Design review of the part built by this model. Coordinates are the model's own, in mm. Face numbers are marked on the shaded views. A direction names the side the tool comes from. Coordinates: 2 decimals unless noted, no trailing zeros. Order: outer loops, then holes, each group sorted by start corner. A loop starts at its lowest first (then second) coordinate and runs counter-clockwise, first axis right, second up. Notation, with made-up numbers: (17, 73.5) - (75, 73.5) arc R20 cw to (75, 93.5) - close; hole circle Ø1 at (80.5, 21). An arc over 180 degrees is marked (long way). Write item = value, one per line. Start each with the question number.
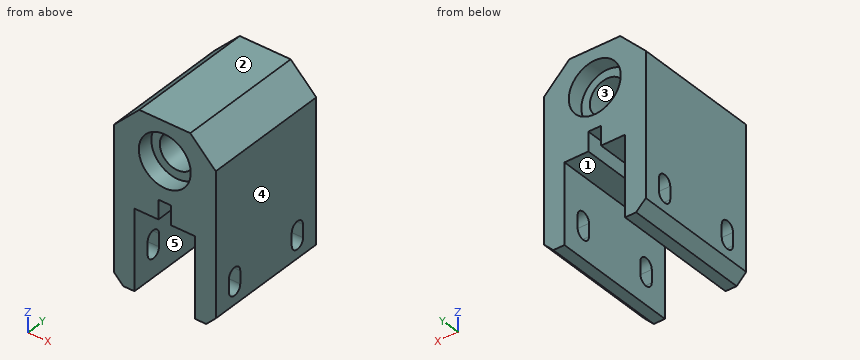
```python
from build123d import *

# Parameters (mm, degrees)
SKETCH1_R           = 5.5
BOSS_EXTRUDE1_DEPTH = 20
SKETCH2_R           = 8.15
CUT_EXTRUDE1_DEPTH  = 5
CUT_EXTRUDE2_DEPTH  = 58.586890869


with BuildPart() as part:
    # Sketch1 → Boss-Extrude1 (new, symmetric)
    with BuildSketch(Plane(origin=(0, 0, 0), x_dir=(1, 0, 0), z_dir=(0, 1, 0))):
        Polygon((-9.5, 43.5), (-9.5, 18.5), (-2, 18.5), (-2, 12.5), (2, 12.5), (2, 18.5), (9.5, 18.5), (9.5, 43.5), (13, 43.5), (16, 40.5), (16, -4), (8, -12), (-8, -12), (-16, -4), (-16, 40.5), (-13, 43.5), align=None)
        with Locations(Location((0, 0, 0), (0, 0, 270))):
            Circle(SKETCH1_R, mode=Mode.SUBTRACT)
    extrude(amount=BOSS_EXTRUDE1_DEPTH, both=True)

    # Sketch2 → Cut-Extrude1 (cut)
    with BuildSketch(Plane(origin=(0, 20, 0), x_dir=(1, 0, 0), z_dir=(0, 1, 0))):
        with Locations(Location((0, 0, 0), (0, 0, 270))):
            Circle(SKETCH2_R)
    cut_extrude1 = extrude(amount=-CUT_EXTRUDE1_DEPTH, mode=Mode.SUBTRACT)

    # Mirror1: Cut-Extrude1 across plane
    add(cut_extrude1.mirror(Plane.ZX), mode=Mode.SUBTRACT)

    # Sketch3 → Cut-Extrude2 (cut, through all)
    with BuildSketch(Plane(origin=(16, 0, 0), x_dir=(0, 0, -1), z_dir=(1, 0, 0))):
        with BuildLine():
            Line((35.5, 10.25), (31.5, 10.25))
            ThreePointArc((31.5, 10.25), (29.25, 12.5), (31.5, 14.75))
            Line((31.5, 14.75), (35.5, 14.75))
            ThreePointArc((35.5, 14.75), (37.75, 12.5), (35.5, 10.25))
        make_face()
        with BuildLine():
            Line((35.5, -14.75), (31.5, -14.75))
            ThreePointArc((31.5, -14.75), (29.25, -12.5), (31.5, -10.25))
            Line((31.5, -10.25), (35.5, -10.25))
            ThreePointArc((35.5, -10.25), (37.75, -12.5), (35.5, -14.75))
        make_face()
    extrude(amount=-CUT_EXTRUDE2_DEPTH, mode=Mode.SUBTRACT)


solid = part.part
```
Item 1: Add section B-B on z = -21. Give the boundary of the cut face in (x, y).
Item 2: Mouldability with a two-part tool opening along Z and no side actions: class the marked faces 1, 2 and 3 as +Z half, -Z half, draft (parallel to the pull), parting line (faces both ways), or undercut.
Item 3: For line 1 (X direction, y = -18.7, z = 0); line 2 (X direction, y = 4.25, z = 0); line 3 (Z direction, x = -12, y = 16), list the stretches that pass through material, from the lowest coordinate up.
Item 4: Add section A-A on y = 12.5. Give the boundary of the cut face in (x, z).
Item 5: Add section D-D on x = 12. Give the boundary of the cut face in (y, z).
Item 6: Add section C-C on x = 0. Give the boundary of the cut face in (y, z), plus the area to 3 significant figures.
Item 7: For P1, Ø6, axis at x = -7, y = -8, coming from the -Z side; P2, Ø5, axis at x = 6.5, y = 5, coming from the -Z side; P3, Ø2, axis at x = 0, y = -10, coming from the -Z side, all flat-tipped, find the tip position at first contact; note any pin that passes through.
Item 8: For the marked faces 4 and 5, list the 3-axis set-ups (+Z, -Z, +X, -X, +Y, -Y) from which the entire face can be reached by the end or side of a thin tool; tool diameter is ignored.
Worked out:
q1.outline = (-16, -20) - (-9.5, -20) - (-9.5, 20) - (-16, 20) - close; (9.5, -20) - (16, -20) - (16, 20) - (9.5, 20) - close
q2.face_1 = -Z half
q2.face_2 = +Z half
q2.face_3 = undercut
q3.line_1 = -16 to -8.15, 8.15 to 16
q3.line_2 = -16 to -5.5, 5.5 to 16
q3.line_3 = -43.5 to 8
q4.outline = (-16, -40.5) - (-13, -43.5) - (-9.5, -43.5) - (-9.5, -37.75) - (-16, -37.75) - close; (-16, -29.25) - (-9.5, -29.25) - (-9.5, -18.5) - (-2, -18.5) - (-2, -12.5) - (2, -12.5) - (2, -18.5) - (9.5, -18.5) - (9.5, -29.25) - (16, -29.25) - (16, 4) - (8, 12) - (-8, 12) - (-16, 4) - close; (9.5, -43.5) - (13, -43.5) - (16, -40.5) - (16, -37.75) - (9.5, -37.75) - close; hole circle Ø11 at (0, 0)
q5.outline = (-20, -43.5) - (20, -43.5) - (20, 8) - (-20, 8) - close; hole (-14.75, -35.5) arc R2.25 ccw to (-10.25, -35.5) - (-10.25, -31.5) arc R2.25 ccw to (-14.75, -31.5) - close; hole (10.25, -35.5) arc R2.25 ccw to (14.75, -35.5) - (14.75, -31.5) arc R2.25 ccw to (10.25, -31.5) - close
q6.outline = (-20, -12.5) - (20, -12.5) - (20, -8.15) - (15, -8.15) - (15, -5.5) - (-15, -5.5) - (-15, -8.15) - (-20, -8.15) - close; (-20, 8.15) - (-15, 8.15) - (-15, 5.5) - (15, 5.5) - (15, 8.15) - (20, 8.15) - (20, 12) - (-20, 12) - close
q6.area = 487 mm2
q7.P1 = -43.5
q7.P2 = -18.5
q7.P3 = -12.5
q8.face_4 = +Z, -Z, +X, +Y, -Y
q8.face_5 = -Z, +Y, -Y
